Could you check a few things on this model? Use its own coordinates, in mm. A direction names the side the tool comes from. Give positions to 0.01 mm unless a question says otherwise; leave off trailing zeros. Order: outer loops, then holes, each group sorted by start corner. A loop starts at its lowest first (then second) coordinate and runs counter-clockwise, first axis right, second up. Notation, with made-up numbers: M 64,-10 L 84,-10 A8 cw 84,-1 Z; hole C 78,31.5 d4. An arc over 180 degrees is marked long. Use a Markdown table: item, result. Add a question column.
```python
from build123d import *

# Parameters (mm, degrees)
SKETCH_W        = 280
SKETCH_H        = 170
PAD_DEPTH       = 6
SKETCH001_R     = 1.7
SKETCH001_W     = 10
SKETCH001_H     = 10
POCKET_DEPTH    = 661.244466
SKETCH002_R     = 1.7
SKETCH002_R_2   = 11.5
POCKET001_DEPTH = 6.001


with BuildPart() as part:
    # Sketch → Pad (new body)
    with BuildSketch(Plane.XY):
        Rectangle(SKETCH_W, SKETCH_H)
    extrude(amount=PAD_DEPTH)

    # Sketch001 (on Face6 of Pad) → Pocket (cut, through all)
    with BuildSketch(Plane.XY.offset(6)):
        with Locations((-135, 60)):
            Circle(SKETCH001_R)
        with Locations((135, 60)):
            Circle(SKETCH001_R)
        with Locations((-135, 80)):
            Rectangle(SKETCH001_W, SKETCH001_H)
        with Locations((135, 80)):
            Rectangle(SKETCH001_W, SKETCH001_H)
    pocket = extrude(amount=-POCKET_DEPTH, mode=Mode.SUBTRACT)

    # Mirrored: Pocket across Sketch001 H_Axis
    add(pocket.mirror(Plane(origin=(0, 0, 6), x_dir=(0, 0, 1), z_dir=(0, 1, 0))), mode=Mode.SUBTRACT)

    # Sketch002 (on Face4 of Mirrored) → Pocket001 (cut, through all)
    with BuildSketch(Plane.XY.offset(6)):
        with Locations((-15.5, -48.35)):
            Circle(SKETCH002_R)
        with Locations((15.5, -48.35)):
            Circle(SKETCH002_R)
        with Locations((15.5, -79.35)):
            Circle(SKETCH002_R)
        with Locations((-15.5, -79.35)):
            Circle(SKETCH002_R)
        with Locations((0, -63.85)):
            Circle(SKETCH002_R_2)
    extrude(amount=-POCKET001_DEPTH, mode=Mode.SUBTRACT)


solid = part.part
```
1) Suppose I cut it at A-A on x = 0. Please give me the cut outline in (y, z).
2) Suppose I cut it at B-B on z = 1.8. Count the separate pieces of the cut face and the enclosed holes in it, and give its area (3 significant figures).
3) For pin 1 (2 mm diameter, centred on x = 15.5, y = -79.35, fed in from +Z); pin 2 (3 mm diameter, centred on x = 133.5, z = 2.5, fed in from -Y); pin 3 (1.8 mm diameter, centred on x = -133, z = 3.5, fed in from +Y); pin 4 (3 mm diameter, centred on y = 82.5, z = 2, fed in from +X), each with a flat end and sliding along its axis, tell me the tip position at first contact or that it passes through.
4) We'd pull the mould along Y, two halves only. Please class faces 1 (the face through (-1.5, -52.45, 3.04)), 2 (the face through (-130, -80, 3)), 3 (the face through (-135, 75, 3)), 4 (the face through (135, -75, 3)): pulls with the +Y half, pulls with the -Y half, needs draft (parallel to the pull), parting line crosses it, or undercut.
5) Please list where these lines run through material, in increasing order: line 1 (Y direction, x = 135, z = 4.3); line 2 (Y direction, x = -15.5, z = 3.9); line 3 (X direction, y = -58.5, z = 0.5). Write a range as from..to.
6) For faces 5 (the face through (-130, 80, 3)), 6 (the face through (130, 80, 3)), 7 (the face through (-140, -1, 3)), 8 (the face through (-135, -75, 3)), 9 (the face through (130, -80, 3)), which set-ups out of +Z, -Z, +X, -X, +Y, -Y let a thin tool reach every point of the face, with its end or its side?
Values found:
| question | item | result |
|---|---|---|
| 1 | outline | M -85,0 L -75.35,0 L -75.35,6 L -85,6 Z; M -52.35,0 L 85,0 L 85,6 L -52.35,6 Z |
| 2 | separate pieces | 1 |
| 2 | enclosed holes | 9 |
| 2 | area | 46,700 mm^2 |
| 3 | pin 1 | passes through |
| 3 | pin 2 | stops at y = -75 |
| 3 | pin 3 | stops at y = 75 |
| 3 | pin 4 | stops at x = 130 |
| 4 | face 1 | undercut |
| 4 | face 2 | needs draft |
| 4 | face 3 | pulls with the +Y half |
| 4 | face 4 | pulls with the -Y half |
| 5 | line 1 | y = -75..-61.7, -58.3..58.3, 61.7..75 |
| 5 | line 2 | y = -85..-81.05, -77.65..-50.05, -46.65..85 |
| 5 | line 3 | x = -140..-135.8, -134.2..-10.18, 10.18..134.2, 135.8..140 |
| 6 | face 5 | +Z, -Z, -X, +Y |
| 6 | face 6 | +Z, -Z, +X, +Y |
| 6 | face 7 | +Z, -Z, -X, +Y, -Y |
| 6 | face 8 | +Z, -Z, -X, -Y |
| 6 | face 9 | +Z, -Z, +X, -Y |
